```python
from build123d import *

# Parameters (mm, degrees)
SKETCH1_W               = 40
SKETCH1_H               = 57.5
SKETCH1_R               = 10.3
SKETCH1_R_2             = 5.925
SKETCH1_R_3             = 1.5
BOSS_EXTRUDE1_DEPTH     = 8
SKETCH1_3_W             = 2
SKETCH1_3_H             = 57.5
BOSS_EXTRUDE2_DEPTH     = 2
SKETCH1_4_R             = 10.3
BOSS_EXTRUDE3_DEPTH     = 4
BOSS_EXTRUDE4_START     = 1
SKETCH1_5_R             = 5.925
SKETCH1_5_R_2           = 1.5
BOSS_EXTRUDE4_DEPTH     = 1
CUT_EXTRUDE1_START      = -6
SKETCH2_R               = 1.9
SKETCH2_R_2             = 1.5
CUT_EXTRUDE1_DEPTH      = 6
SKETCH3_W               = 0.4
SKETCH3_H               = 20.6
SKETCH3_W_2             = 20.6
SKETCH3_H_2             = 0.4
CUT_EXTRUDE_THIN1_DEPTH = 3


with BuildPart() as part:
    # Sketch1 → Boss-Extrude1 (new body)
    # profile 1 of 3: a face of its own
    with BuildSketch(Plane(origin=(0, 0, 0), x_dir=(1, 0, 0), z_dir=(0, 1, 0))):
        with Locations((5, 18.75)):
            Rectangle(SKETCH1_W, SKETCH1_H)
        with Locations((0, 22.5)):
            Circle(SKETCH1_R, mode=Mode.SUBTRACT)
        Circle(SKETCH1_R_2, mode=Mode.SUBTRACT)
    # profile 2 of 3: a face of its own
    with BuildSketch(Plane(origin=(0, 0, 0), x_dir=(1, 0, 0), z_dir=(0, 1, 0))):
        with Locations((0, 22.5)):
            Circle(SKETCH1_R)
    # profile 3 of 3: a face of its own
    with BuildSketch(Plane(origin=(0, 0, 0), x_dir=(1, 0, 0), z_dir=(0, 1, 0))):
        Circle(SKETCH1_R_2)
        with Locations(Location((-4.35, 0, 0), (0, 0, 270))):
            Circle(SKETCH1_R_3, mode=Mode.SUBTRACT)
        with Locations(Location((4.35, 0, 0), (0, 0, 270))):
            Circle(SKETCH1_R_3, mode=Mode.SUBTRACT)
    extrude(amount=-BOSS_EXTRUDE1_DEPTH)

    # Sketch1_3 → Boss-Extrude2 (add)
    with BuildSketch(Plane(origin=(0, 0, 0), x_dir=(1, 0, 0), z_dir=(0, 1, 0))):
        with Locations((-16, 18.75)):
            Rectangle(SKETCH1_3_W, SKETCH1_3_H)
        with Locations((26, 18.75)):
            Rectangle(SKETCH1_3_W, SKETCH1_3_H)
    extrude(amount=-BOSS_EXTRUDE2_DEPTH)

    # Sketch1_4 → Boss-Extrude3 (add)
    with BuildSketch(Plane(origin=(0, 0, 0), x_dir=(1, 0, 0), z_dir=(0, 1, 0))):
        with Locations(Location((0, 22.5, 0), (0, 0, 270))):
            Circle(SKETCH1_4_R)
    extrude(amount=BOSS_EXTRUDE3_DEPTH)

    # Sketch1_5 → Boss-Extrude4 (add)
    with BuildSketch(Plane(origin=(0, 0, 0), x_dir=(1, 0, 0), z_dir=(0, 1, 0)).offset(BOSS_EXTRUDE4_START)):
        with Locations(Location((0, 0, 0), (0, 0, 270))):
            Circle(SKETCH1_5_R)
        with Locations(Location((-4.35, 0, 0), (0, 0, 270))):
            Circle(SKETCH1_5_R_2, mode=Mode.SUBTRACT)
        with Locations(Location((4.35, 0, 0), (0, 0, 270))):
            Circle(SKETCH1_5_R_2, mode=Mode.SUBTRACT)
    extrude(amount=-BOSS_EXTRUDE4_DEPTH)

    # Sketch2 → Cut-Extrude1 (cut)
    # profile 1 of 2: a face of its own
    with BuildSketch(Plane.XZ.offset(8).offset(CUT_EXTRUDE1_START)):
        with Locations(Location((-4.35, 0, 0), (0, 0, 270))):
            Circle(SKETCH2_R)
        with Locations(Location((-4.35, 0, 0), (0, 0, 90))):
            Circle(SKETCH2_R_2, mode=Mode.SUBTRACT)
    # profile 2 of 2: a face of its own
    with BuildSketch(Plane.XZ.offset(8).offset(CUT_EXTRUDE1_START)):
        with Locations(Location((4.35, 0, 0), (0, 0, 270))):
            Circle(SKETCH2_R)
        with Locations(Location((4.35, 0, 0), (0, 0, 90))):
            Circle(SKETCH2_R_2, mode=Mode.SUBTRACT)
    extrude(amount=CUT_EXTRUDE1_DEPTH, mode=Mode.SUBTRACT)

    # Sketch3 → Cut-Extrude-Thin1 (cut)
    with BuildSketch(Plane(origin=(0, 4, 0), x_dir=(1, 0, 0), z_dir=(0, 1, 0))):
        with Locations((0, 22.5)):
            Rectangle(SKETCH3_W, SKETCH3_H)
        with Locations((0, 22.5)):
            Rectangle(SKETCH3_W_2, SKETCH3_H_2)
    extrude(amount=-CUT_EXTRUDE_THIN1_DEPTH, mode=Mode.SUBTRACT)


solid = part.part
```
Check sheet for the modelled part. Datum: model origin and axes. Units: mm. A direction names the side the tool comes from. Coordinates: 2 decimals unless noted, no trailing zeros. Order: outer loops, then holes, each group sorted by start corner. A loop starts at its lowest first (then second) coordinate and runs counter-clockwise, first axis right, second up. Notation, with made-up numbers: (-9, 47.5) -> (8, 47.5) arc R17 cw to (8, 51.5) -> close; hole circle Ø2 at (78.25, -10). An arc over 180 degrees is marked (long way). Write item = value, one per line. Start each with the question number.
1) Mould release check, pull along Z, two halves, no side actions. Record for faces 1 (the cylindrical face through (-5.814, -0.479, -0.325)), 2 (the flat face through (-0.2, 3, -17)), 3 (the flat face through (5, -4, 10)): +Z half, -Z half, draft (parallel to the pull), parting line (faces both ways), or undercut.
2) Material ranges on L1, parallel to X at y = -0.2, z = 0; L2, parallel to X at y = -6.8, z = 0; L3, parallel to Z at x = -4.35, y = -0.8, recorded low to high.
3) Cross-section at C-C (x = 4.35). Enter the section's corners in (y, z), then the cut area to 3 significant figures.
4) Go/stop test with flat-tipped pins: P1, Ø0.9, axis at x = 4.5, y = 3, coming from the -Z side; P2, Ø0.9, axis at x = -3, y = 3, coming from the +Z side; P3, Ø3.5, axis at x = -4.35, z = 0, coming from the +Y side. Record where each tip stops, or that it passes through.
5) Cross-section at A-A (y = 1.75). Enter the section's corners in (x, z), then the cut area to 3 significant figures.
6) Access from +Z, -Z, +X, -X, +Y, -Y to the whole of each face (thin tool, end or side, straight path). Record for faces 4 (the flat face through (25, -5, -18)), 5 (the flat face through (-16, -2, -19)), 6 (the flat face through (0, 1, 0)), 7 (the cylindrical face through (-6.205, -4.958, 0.412)), 8 (the cylindrical face through (3.094, 1.972, -12.676)).
7) Cross-section at D-D (z = -40.5). Enter the section's corners in (x, y), then the cut area to 3 significant figures.
8) Cross-section at B-B (z = 0). Enter the section's corners in (x, y) (3 decimals), then the cut area to 3 significant figures.
Ans:
q1.face_1 = undercut
q1.face_2 = draft
q1.face_3 = +Z half
q2.L1 = -17 to -5.85, -2.85 to 2.85, 5.85 to 27
q2.L2 = -15 to -6.25, -2.45 to 2.45, 6.25 to 25
q2.L3 = -47.5 to -1.5, 1.5 to 10
q3.outline = (-8, -47.5) -> (0, -47.5) -> (0, -31.84) -> (4, -31.84) -> (4, -22.7) -> (1, -22.7) -> (1, -22.3) -> (4, -22.3) -> (4, -13.16) -> (0, -13.16) -> (0, -4.02) -> (1, -4.02) -> (1, -1.5) -> (-2, -1.5) -> (-2, -1.9) -> (-8, -1.9) -> close; (-8, 1.9) -> (-2, 1.9) -> (-2, 1.5) -> (1, 1.5) -> (1, 4.02) -> (0, 4.02) -> (0, 10) -> (-8, 10) -> close
q3.area = 510 mm²
q4.P1 = -31.97
q4.P2 = -12.52
q4.P3 = 1
q5.outline = (-10.3, -22.7) arc R10.3 ccw to (-0.2, -32.8) -> (-0.2, -22.7) -> close; (-10.3, -22.3) -> (-0.2, -22.3) -> (-0.2, -12.2) arc R10.3 ccw to start; (0.2, -32.8) arc R10.3 ccw to (10.3, -22.7) -> (0.2, -22.7) -> close; (0.2, -22.3) -> (10.3, -22.3) arc R10.3 ccw to (0.2, -12.2) -> close
q5.area = 317 mm²
q6.face_4 = +Z, -Z, +X, -Y
q6.face_5 = +Z, -Z, -X, -Y
q6.face_6 = +Z, +X, -X, +Y
q6.face_7 = -Y
q6.face_8 = +Y
q7.outline = (-17, -2) -> (-15, -2) -> (-15, -8) -> (25, -8) -> (25, -2) -> (27, -2) -> (27, 0) -> (-17, 0) -> close
q7.area = 328 mm²
q8.outline = (-17, -2) -> (-15, -2) -> (-15, -8) -> (-6.25, -8) -> (-6.25, -2) -> (-5.85, -2) -> (-5.85, 1) -> (-5.925, 1) -> (-5.925, 0) -> (-17, 0) -> close; (-2.85, -2) -> (-2.45, -2) -> (-2.45, -8) -> (2.45, -8) -> (2.45, -2) -> (2.85, -2) -> (2.85, 1) -> (-2.85, 1) -> close; (5.85, -2) -> (6.25, -2) -> (6.25, -8) -> (25, -8) -> (25, -2) -> (27, -2) -> (27, 0) -> (5.925, 0) -> (5.925, 1) -> (5.85, 1) -> close
q8.area = 276 mm²
